Could you check a few things on this drawing? It's one solid part, dimensions in mm from its lowest x, y, z. Give positions to 0.01 mm unless a question says otherwise; leave off trailing zeros. Order: outer loops, then holes, each group sorted by start corner. A loop starts at its lowest first (then second) coordinate and runs counter-clockwise, first axis right, second up. Notation, with made-up numbers: (63, 10) -> (76, 10) arc R32 cw to (76, 48) -> close; hole circle Ø8 at (50, -28.5). An arc over 180 degrees is marked (long way). Write each question's results on one line, items separated by ' | '.
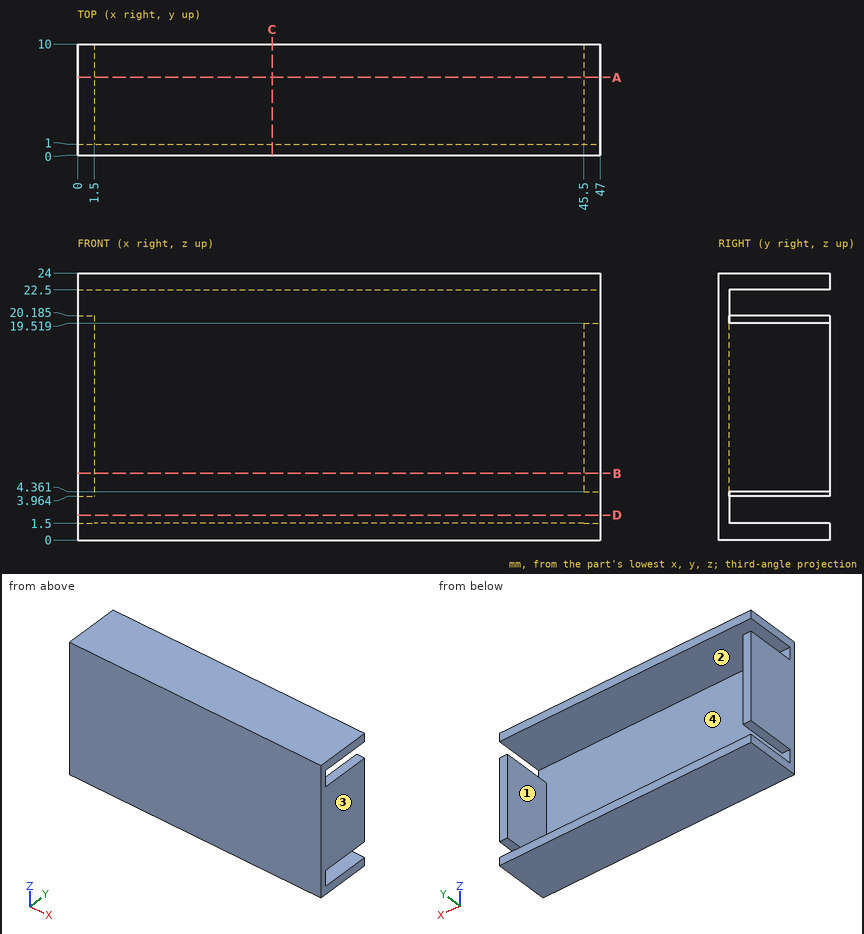
Q1. Suppose I cut it at B-B on z = 6. Please give me the cut outline in (x, y).
Here are the results:
outline: (0, 0) -> (47, 0) -> (47, 10) -> (45.5, 10) -> (45.5, 1) -> (1.5, 1) -> (1.5, 10) -> (0, 10) -> close
Q2. Suppose I cut it at A-A on y = 7. Please give me the cut outline in (x, z) (1 decimal).
Here are the results:
outline: (0, 0) -> (47, 0) -> (47, 1.5) -> (0, 1.5) -> close; (0, 4) -> (1.5, 4) -> (1.5, 20.2) -> (0, 20.2) -> close; (0, 22.5) -> (47, 22.5) -> (47, 24) -> (0, 24) -> close; (45.5, 4.4) -> (47, 4.4) -> (47, 19.5) -> (45.5, 19.5) -> close
Q3. I'm going to push a flat-ended pin straight in: pin 1 Ø12 at (x, z) = (31.5, 10) entering from +Y. Where does the tip first touch, or does it pass through?
Here are the results:
pin 1: stops at y = 1
Q4. Suppose I cut it at D-D on z = 2.25. Please give me the cut outline in (x, y).
Here are the results:
outline: (0, 0) -> (47, 0) -> (47, 1) -> (0, 1) -> close
Q5. Suppose I cut it at C-C on x = 17.5. Please give me the cut outline in (y, z).
Here are the results:
outline: (0, 0) -> (10, 0) -> (10, 1.5) -> (1, 1.5) -> (1, 22.5) -> (10, 22.5) -> (10, 24) -> (0, 24) -> close
Q6. Thinking about a two-plate mould opening in X: for the marked faces 1, 2, 3 and 4, which applies, +X half, -X half, draft (parallel to the pull), parting line (faces both ways), or undercut?
Here are the results:
face 1: undercut | face 2: draft | face 3: +X half | face 4: undercut
Q7. I need wall thicknesses on line 1 along Z through (x, y) = (27.5, 6.75); line 2 along X through (y, z) = (3.25, 10); line 3 along Y through (x, z) = (22.5, 11.75). Which ranges of each line are inside material? Lowest first, please.
Here are the results:
line 1: z = 0 to 1.5, 22.5 to 24 | line 2: x = 0 to 1.5, 45.5 to 47 | line 3: y = 0 to 1
